Autodesk Inventor part; units mm, degrees
ref_plane "YZ Plane" through (0, 0, 0) normal (1, 0, 0) x (0, 1, 0)
ref_plane "XZ Plane" through (0, 0, 0) normal (0, 1, 0) x (-1, 0, 0)
ref_plane "XY Plane" through (0, 0, 0) normal (0, 0, 1) x (1, 0, 0)
sketch "Sketch1" plane through (0, 0, 0) normal (0, 0, 1) x (1, 0, 0)
  line L0 (-11.5, -75) -> (11.5, -75)
  line L1 (11.5, -75) -> (11.5, 75)
  line L2 (11.5, 75) -> (-11.5, 75)
  line L3 (-11.5, 75) -> (-11.5, -75)
  line L4 (-11.5, -75) -> (11.5, 75) construction
  line L5 (11.5, -75) -> (-11.5, 75) construction
  line L6 (11.5, 75) -> (4.5, 75)
  line L7 (4.5, 75) -> (4.5, -5)
  line L8 (4.5, -5) -> (11.5, -5)
  line L9 (11.5, -5) -> (11.5, 75)
  point P0 (0, 0)
  dimension "key_width" = 23
  dimension "key_length" = 150
  dimension "blackkey_length" = 80
  dimension "blackkey_halfwidth" = 7
extrude "Extrusion1" add sketch "Sketch1" against normal blind 20 contours L3 L2 L7 L8 L1 L0
chamfer "Chamfer1" distance 1 angle 45 5 edges at (11.5, -40, 0) (0, -75, 0) (-11.5, 0, 0) (4.5, 35, 0) (8, -5, 0)
properties part number "key1"
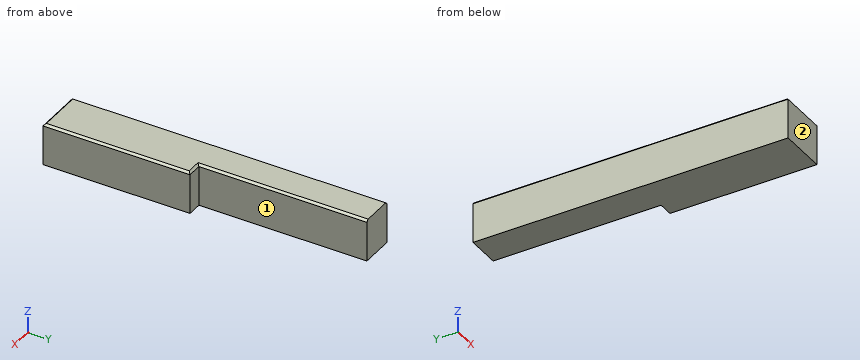
Work out the finished part from the listing and answer in its coordinate system (mm). Face numbers are marked on the shaded views. A direction names the side the tool comes from. Give positions to 0.01 mm unless a question says otherwise; leave off trailing zeros. Loops run counter-clockwise (first coordinate to the right, second up) from the corner with the lowest first, then second, coordinate; pieces in that order, holes last. Notation, with made-up numbers: M 68.25,-10 L 84.25,-10 A23 ccw 84.25,0 Z; hole C 69,5 d8. An arc over 180 degrees is marked long. One line per item, written item: value. Start each with the question number.
1. Find section A-A (z = -17). Give the vertices of the cut face in (x, y).
2. Find section B-B (y = 3). Give the vertices of the cut face in (x, z).
3. Which of the six approach directions +Z, -Z, +X, -X, +Y, -Y give full straight-line access (tool end or side, diameter ignored) to the marked faces 1 and 2?
4. Each of these flat-tipped pins is pushed along its axis until it touches: P1, Ø3.5, axis at x = 9.5, z = -12.5, coming from the +Y side; P2, Ø2, axis at y = 52, z = -14.5, coming from the +X side. Where does it stop, or does it pass through?
5. Find the intervals of material crossed by probe 1 along Y at (x, z) = (10, -12.25); probe 2 along X at (y, z) = (27, -7.25), in increasing order.
Reported:
1. outline: M -11.5,-75 L 11.5,-75 L 11.5,-5 L 4.5,-5 L 4.5,75 L -11.5,75 Z
2. outline: M -11.5,-20 L 4.5,-20 L 4.5,-1 L 3.5,0 L -10.5,0 L -11.5,-1 Z
3. face 1: +Z, -Z, +X, +Y
3. face 2: +Z, -Z, +X, -X, -Y
4. P1: stops at y = -5
4. P2: stops at x = 4.5
5. probe 1: y = -75 to -5
5. probe 2: x = -11.5 to 4.5
